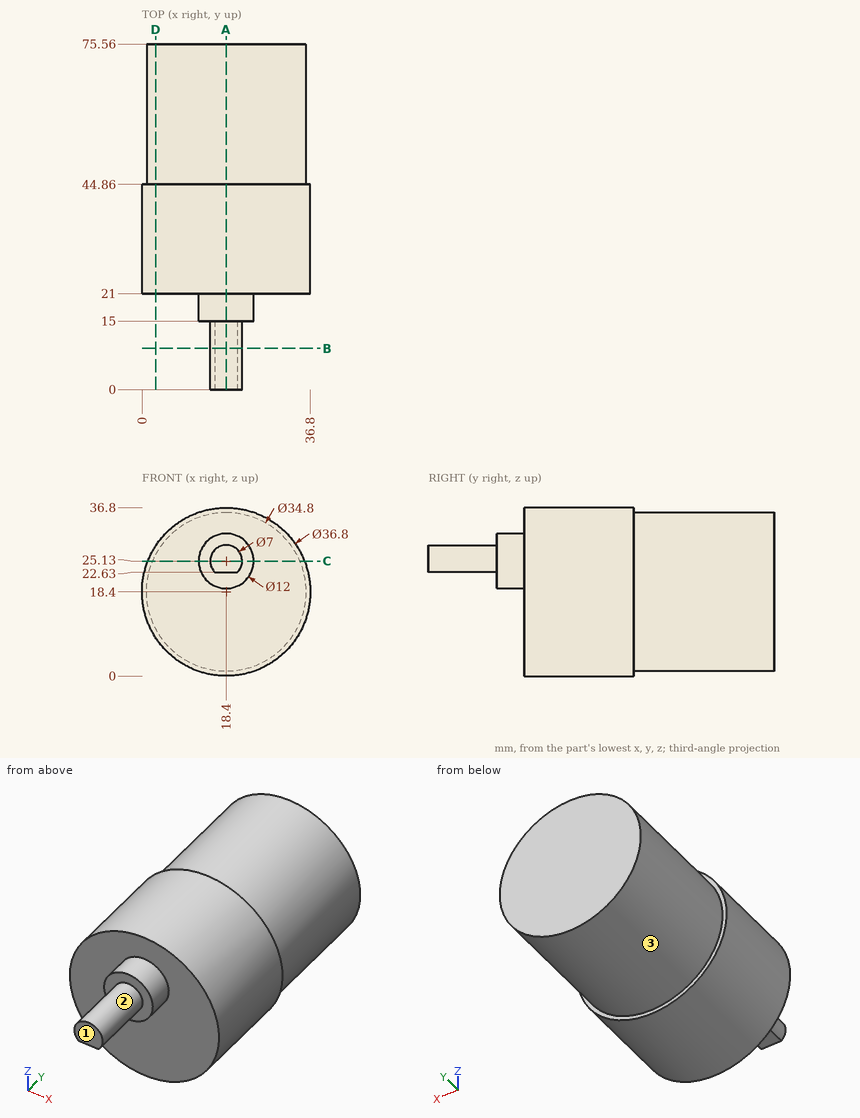
Job drawing, mm, ordinate dimensions from the low corner. One solid piece. A direction names the side the tool comes from. Round coordinates to 2 decimals unless told otherwise and drop trailing zeros. Order: outer loops, then holes, each group sorted by start corner. A loop starts at its lowest first (then second) coordinate and runs counter-clockwise, first axis right, second up. Notation, with made-up numbers: (-31.5, 50.5) -> (13.5, 50.5) arc R7 cw to (13.5, 58.5) -> close; hole circle Ø5 at (77, 21.5). An arc over 180 degrees is marked (long way). Write item = value, one per line.
(1) 3-axis set-ups, long thin cutter, end or side, ignore diameter. For the marked faces 1, 2 and 3: which of +Z, -Z, +X, -X, +Y, -Y reach the whole face in a straight line?
Answers follow:
face_1 = +Z, -Z, +X, -X, -Y
face_2 = -Y
face_3 = +Y
(2) Flat gauge pins, fed straight in: P1, Ø8, axis at y = 45, z = 22, coming from the -X side; P2, Ø1, axis at y = 38, z = 7.5, coming from the +X side; P3, Ø2, axis at x = 12.5, y = 46.5, coming from the +Z side; P4, Ø4, axis at x = 11.5, y = 8.5, coming from the +Z side. Where does each tip first touch, or does it go through?
Answers follow:
P1 = 0
P2 = 33.58
P3 = 35.1
P4 = through
(3) Cut at C-C (z = 25.13). Write the cut outline in (x, y).
Answers follow:
outline = (1.27, 21) -> (12.4, 21) -> (12.4, 15) -> (14.9, 15) -> (14.9, 0) -> (21.9, 0) -> (21.9, 15) -> (24.4, 15) -> (24.4, 21) -> (35.53, 21) -> (35.53, 44.86) -> (34.45, 44.86) -> (34.45, 75.56) -> (2.35, 75.56) -> (2.35, 44.86) -> (1.27, 44.86) -> close
(4) Cut at B-B (y = 9). Write the cut outline in (x, z), plus the area to 3 significant figures.
Answers follow:
outline = (15.95, 22.63) -> (20.85, 22.63) arc R3.5 ccw (long way) to start
area = 35.1 mm²
(5) Cut at A-A (x = 18.4). Write the cut outline in (y, z), plus the area to 3 significant figures.
Answers follow:
outline = (0, 22.63) -> (15, 22.63) -> (15, 19.13) -> (21, 19.13) -> (21, 0) -> (44.86, 0) -> (44.86, 1) -> (75.56, 1) -> (75.56, 35.8) -> (44.86, 35.8) -> (44.86, 36.8) -> (21, 36.8) -> (21, 31.13) -> (15, 31.13) -> (15, 28.63) -> (0, 28.63) -> close
area = 2,110 mm²
(6) Cut at D-D (x = 3). Write the cut outline in (y, z), plus the area to 3 significant figures.
Answers follow:
outline = (21, 8.33) -> (44.86, 8.33) -> (44.86, 10.3) -> (75.56, 10.3) -> (75.56, 26.5) -> (44.86, 26.5) -> (44.86, 28.47) -> (21, 28.47) -> close
area = 978 mm²
(7) Drill centre lines: L1, parallel to Y at x = 33.5, z = 13.5; L2, parallel to Z at x = 16, y = 58.5; L3, parallel to Z at x = 22.5, y = 70.5. Where is each one in solid material? Low to high.
Answers follow:
L1 = 21 to 75.56
L2 = 1.17 to 35.63
L3 = 1.49 to 35.31
